Here's how the part is built. I have some questions about the finished solid (model axes, mm). A direction names the side the tool comes from. Give positions to 0.01 mm unless a question says otherwise; leave off trailing zeros. Loops run counter-clockwise (first coordinate to the right, second up) from the corner with the lowest first, then second, coordinate; pieces in that order, holes last.
Q1. If we section it at B-B (x = 0): Please give me the cut outline in (y, z), plus the area to 3 significant figures.
Q2. If we section it at A-A (y = 0): Please give me the cut outline in (x, z).
Q3. Will these pins go through, and if not, where does the flat tip stop? P1, Ø20, axis at x = 0, z = 23.5, coming from the +Y side; P2, Ø7.5, axis at y = -0.5, z = 16.5, coming from the +X side; P3, Ø2, axis at y = 1.5, z = 15.5, coming from the -X side.
Q4. For faces 1 (the face through (-2.71, -29.014, 11.297)), 2 (the face through (0, -26, 18)), 3 (the face through (0, 26, 18)), which set-ups out of +Z, -Z, +X, -X, +Y, -Y let a thin tool reach every point of the face, with its end or its side?
Q5. If we section it at D-D (z = 23.5): Give the number of separate pieces and of enclosed holes in the cut face, plus the area to 3 significant figures.
Q6. We'd pull the mould along X, two halves only. Please class faces 4 (the face through (-7, 30, 12)), 5 (the face through (0, 26.5, 36)), 6 (the face through (-26, 0, 18)): +X half, -X half, draft (parallel to the pull), parting line (faces both ways), or undercut.
Q7. I need wall thicknesses on line 1 (X direction, y = -10, z = 39); line 2 (Z direction, x = 0, y = -27); line 3 (X direction, y = -20.5, z = 42). Which ranges of each line are inside material? Lowest first, please.
Q8. If we section it at C-C (x = -21): Please give me the cut outline in (y, z), plus the area to 3 significant figures.
Autodesk Inventor part; units mm, degrees
ref_plane "YZ Plane" through (0, 0, 0) normal (1, 0, 0) x (0, 1, 0)
ref_plane "XZ Plane" through (0, 0, 0) normal (0, 1, 0) x (-1, 0, 0)
ref_plane "XY Plane" through (0, 0, 0) normal (0, 0, 1) x (1, 0, 0)
sketch "Sketch1" plane through (0, 0, 0) normal (0, 0, 1) x (1, 0, 0)
  line L0 (-28, 30) -> (28, 30)
  line L1 (30, 28) -> (30, -28)
  line L2 (28, -30) -> (-28, -30)
  line L3 (-30, -28) -> (-30, 28)
  arc A0 (-28, 30) -> (-30, 28) centre (-28, 28) ccw
  arc A1 (-30, -28) -> (-28, -30) centre (-28, -28) ccw
  arc A2 (28, -30) -> (30, -28) centre (28, -28) ccw
  arc A3 (30, 28) -> (28, 30) centre (28, 28) ccw
  point P0 (0, 0)
  point P1 (-30, 30)
  point P2 (30, -30)
  point P3 (30, 30)
  dimension "d0" = 60
  dimension "d1" = 60
  dimension "d2" = 30
  dimension "d3" = 30
  dimension "d4" = 2
extrude "Extrusion1" add sketch "Sketch1" along normal blind 45
sketch "Sketch2" plane through (0, 0, 45) normal (0, 0, 1) x (1, 0, 0)
  line L0 (-24.5, 26.5) -> (24.5, 26.5)
  line L1 (26.5, 24.5) -> (26.5, -24.5)
  line L2 (24.5, -26.5) -> (-24.5, -26.5)
  line L3 (-26.5, -24.5) -> (-26.5, 24.5)
  arc A0 (-24.5, 26.5) -> (-26.5, 24.5) centre (-24.5, 24.5) ccw
  arc A1 (-26.5, -24.5) -> (-24.5, -26.5) centre (-24.5, -24.5) ccw
  arc A2 (24.5, -26.5) -> (26.5, -24.5) centre (24.5, -24.5) ccw
  arc A3 (26.5, 24.5) -> (24.5, 26.5) centre (24.5, 24.5) ccw
  point P0 (0, 0)
  point P1 (-26.5, 26.5)
  point P2 (26.5, -26.5)
  point P3 (26.5, 26.5)
  dimension "d7" = 53
  dimension "d8" = 53
  dimension "d9" = 26.5
  dimension "d10" = 26.5
  dimension "d11" = 2
extrude "Extrusion2" cut sketch "Sketch2" against normal blind 24.5
sketch "Sketch3" plane through (30, -28, 0) normal (1, 0, 0) x (0, 0, -1)
  circle A0 centre (-23.5, 28) radius 18.5
  line L0 (0, 0) -> (0, 56)
  point P0 (0, 28)
  point P1 (0, 28)
  dimension "d14" = 37
  dimension "d15" = 23.5
extrude "Extrusion3" cut sketch "Sketch3" against normal blind 2
mirror "Mirror1" about plane through (0, 0, 0) normal (1, 0, 0) of "Extrusion3"
sketch "Sketch4" plane through (-28, 30, 0) normal (0, 1, 0) x (1, 0, 0)
  circle A0 centre (28, -23.5) radius 12.5
  point P0 (28, 0)
  dimension "d18" = 25
  dimension "d19" = 23.5
extrude "Extrusion4" cut sketch "Sketch4" against normal blind 2
mirror "Mirror2" about plane through (0, 0, 0) normal (0, 1, 0) of "Extrusion4"
sketch "Sketch5" plane through (-28, 0, 23.5) normal (-1, 0, 0) x (0, 0, 1)
  circle A0 centre (0, 0) radius 9.75
  circle A1 centre (0, 0) radius 18.5
  point P0 (-23.5, 0)
  dimension "d22" = 19.5
extrude "Extrusion5" cut sketch "Sketch5" against normal blind 2 contours A0
pattern_circular "Circular Pattern1" count 4 over 360 about axis through (0, 0, -10) along (0, 0, 1) of "Extrusion5"
sketch "Sketch6" plane through (0, 0, 20.5) normal (0, 0, 1) x (1, 0, 0)
  line L0 (-20, 17) -> (22, 17)
  line L1 (22, 17) -> (22, -20)
  line L2 (22, -20) -> (-20, -20)
  line L3 (-20, -20) -> (-20, 17)
  point P0 (0, 0)
properties part number "sampleChamber_singlePiece_filipeSample_V2"
Check sheet entries:
1. outline: (-30, 0) - (30, 0) - (30, 11) - (28, 11) - (28, 13.75) - (26, 13.75) - (26, 20.5) - (-26, 20.5) - (-26, 13.75) - (-28, 13.75) - (-28, 11) - (-30, 11) - close; (-30, 36) - (-28, 36) - (-28, 33.25) - (-26.5, 33.25) - (-26.5, 45) - (-30, 45) - close; (26.5, 33.25) - (28, 33.25) - (28, 36) - (30, 36) - (30, 45) - (26.5, 45) - close
1. area: 1,240 mm2
2. outline: (-30, 0) - (30, 0) - (30, 5) - (28, 5) - (28, 13.75) - (26, 13.75) - (26, 20.5) - (-26, 20.5) - (-26, 13.75) - (-28, 13.75) - (-28, 5) - (-30, 5) - close; (-30, 42) - (-28, 42) - (-28, 33.25) - (-26.5, 33.25) - (-26.5, 45) - (-30, 45) - close; (26.5, 33.25) - (28, 33.25) - (28, 42) - (30, 42) - (30, 45) - (26.5, 45) - close
3. P1: stops at y = 28
3. P2: stops at x = 28
3. P3: stops at x = -26
4. face 1: -Y
4. face 2: +Z, -Y
4. face 3: +Z, +Y
5. separate pieces: 4
5. enclosed holes: 0
5. area: 426 mm2
6. face 4: draft
6. face 5: undercut
6. face 6: -X half
7. line 1: x = -28 to -26.5, 26.5 to 28
7. line 2: z = 0 to 13.75, 33.25 to 45
7. line 3: x = -30 to -26.5, 26.5 to 30
8. outline: (-30, 0) - (30, 0) - (30, 45) - (26.5, 45) - (26.5, 20.5) - (-26.5, 20.5) - (-26.5, 45) - (-30, 45) - close
8. area: 1,400 mm2
